Could you check a few things on this model? Use its own coordinates, in mm. Face numbers are marked on the shaded views. Give positions to 0.01 mm unless a question says otherwise; leave off trailing zeros. Order: outer loops, then holes, each group sorted by start corner. A loop starts at its lowest first (then second) coordinate and runs counter-clockwise, first axis right, second up. Notation, with made-up numbers: M 24,45.5 L 57,45.5 A23 ccw 57,79.5 Z; hole C -19,43 d9. An arc over 180 degrees is marked long. Answer in a Markdown table with one row per item. Add a question column.
```python
from build123d import *

# Parameters (mm, degrees)
F0_R     = 6.5
F1_DEPTH = 49.2
F2_DEPTH = 32
F3_DEPTH = 41.7


with BuildPart() as f1:
    # F0 (on Front) → F1 (new body)
    with BuildSketch(Plane.XZ):
        with BuildLine():
            Line((24.735266, 68.032924), (18.390851, 76.765262))
            ThreePointArc((18.390851, 76.765262), (-46.398298, 63.861779), (-78.691188, 6.231032))
            Line((-78.691188, 6.231032), (-72.346773, -2.501307))
            ThreePointArc((-72.346773, -2.501307), (-42.549774, 58.56474), (24.735266, 68.032924))
        make_face()
        with BuildLine():
            Line((37.798947, 50.052309), (24.735266, 68.032924))
            ThreePointArc((24.735266, 68.032924), (-42.549774, 58.56474), (-72.346773, -2.501307))
            Line((-72.346773, -2.501307), (-59.283092, -20.481921))
            Line((-59.283092, -20.481921), (-28.170116, 2.122979))
            ThreePointArc((-28.170116, 2.122979), (-16.604933, 22.85473), (6.685972, 27.447409))
            Line((6.685972, 27.447409), (37.798947, 50.052309))
        make_face()
        with Locations((-54.35288, 17.660321)):
            Circle(F0_R, mode=Mode.SUBTRACT)
        with Locations((0, 57.15)):
            Circle(F0_R, mode=Mode.SUBTRACT)
    extrude(amount=F1_DEPTH)

    # F0 (on Front) → F2 (join)
    with BuildSketch(Plane.XZ):
        with BuildLine():
            Line((18.390851, 76.765262), (-49.64947, 170.41473))
            ThreePointArc((-49.64947, 170.41473), (-104.331882, 143.600517), (-146.731509, 99.8805))
            Line((-146.731509, 99.8805), (-78.691188, 6.231032))
            ThreePointArc((-78.691188, 6.231032), (-46.398298, 63.861779), (18.390851, 76.765262))
        make_face()
    extrude(amount=F2_DEPTH)

    # F0 (on Front) → F3 (cut)
    with BuildSketch(Plane.XZ):
        with BuildLine():
            Line((37.798947, 50.052309), (24.735266, 68.032924))
            ThreePointArc((24.735266, 68.032924), (-42.549774, 58.56474), (-72.346773, -2.501307))
            Line((-72.346773, -2.501307), (-59.283092, -20.481921))
            Line((-59.283092, -20.481921), (-28.170116, 2.122979))
            ThreePointArc((-28.170116, 2.122979), (-16.604933, 22.85473), (6.685972, 27.447409))
            Line((6.685972, 27.447409), (37.798947, 50.052309))
        make_face()
        with Locations((-54.35288, 17.660321)):
            Circle(F0_R, mode=Mode.SUBTRACT)
        with Locations((0, 57.15)):
            Circle(F0_R, mode=Mode.SUBTRACT)
    extrude(amount=F3_DEPTH, mode=Mode.SUBTRACT)


solid = f1.part
```
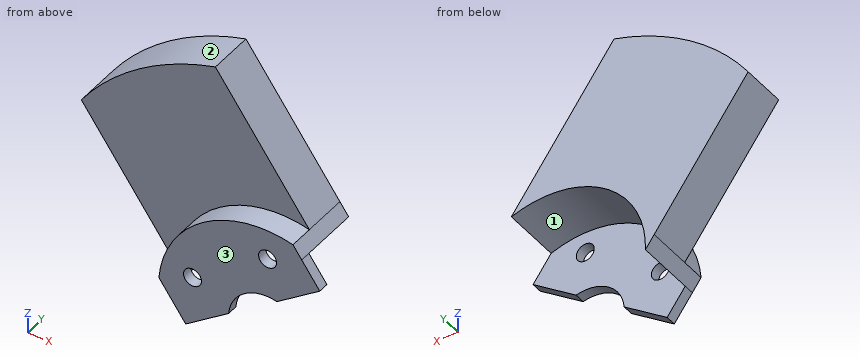
1. If I drill on line 1 along Y through (x, z) = (-79.5, 104.5); line 2 along Y through (x, z) = (-64, 0); line 3 along X through (y, z) = (-44, 57), over which ranges is the centre line in solid material (lowest first)? Write a range as [from, to].
2. Thinking about a two-plate mould opening in X: for the marked faces 1, 2 and 3, which applies, pulls with the +X half, pulls with the -X half, needs draft (parallel to the pull), parting line crosses it, or undercut?
3. Suppose I cut it at D-D on x = -11. List the corners of the cut face in (y, z) for me, plus the area to 3 significant figures.
4. Suppose I cut it at A-A on z = 57.15. List the corners of the cut face in (x, y) for me.
5. Suppose I cut it at B-B on x = -57. List the corners of the cut face in (y, z) for me, plus the area to 3 significant figures.
6. Will these pins go through, and if not, where does the flat tip stop? P1, Ø10, axis at x = -90.5, z = 108.5, coming from the -Y side; P2, Ø12, axis at x = -30.5, y = -8.5, coming from the -Z side; P3, Ø4, axis at x = -126, z = 66.5, coming from the -Y side; P4, Ø3, axis at x = 15, z = 35.5, coming from the +Y side.
7. Suppose I cut it at C-C on y = -28.5. List the corners of the cut face in (x, z) for me, plus the area to 3 significant figures.
Findings below:
| question | item | result |
|---|---|---|
| 1 | line 1 | [-32, 0] |
| 1 | line 2 | [-49.2, -41.7] |
| 1 | line 3 | [-54.61, -6.5], [6.5, 32.75] |
| 2 | face 1 | undercut |
| 2 | face 2 | pulls with the -X half |
| 2 | face 3 | needs draft |
| 3 | outline | M -49.2,26.02 L -41.7,26.02 L -41.7,71.55 L 0,71.55 L 0,117.22 L -32,117.22 L -32,78.17 L -49.2,78.17 Z |
| 3 | area | 1,920 mm2 |
| 4 | outline | M -115.69,-32 L -54.45,-32 L -54.45,-49.2 L -6.5,-49.2 L -6.5,-41.7 L -44.43,-41.7 L -44.43,0 L -115.69,0 Z; M 6.5,-49.2 L 32.64,-49.2 L 32.64,-41.7 L 6.5,-41.7 Z |
| 5 | outline | M -49.2,-18.82 L -41.7,-18.82 L -41.7,11.72 L -49.2,11.72 Z; M -49.2,23.6 L -41.7,23.6 L -41.7,44.62 L 0,44.62 L 0,168.1 L -32,168.1 L -32,54.61 L -49.2,54.61 Z |
| 5 | area | 4,510 mm2 |
| 6 | P1 | y = -32 |
| 6 | P2 | z = 62.51 |
| 6 | P3 | through |
| 6 | P4 | y = -41.7 |
| 7 | outline | M -146.73,99.88 L -72.35,-2.5 A72.39 cw 24.74,68.03 L -49.65,170.41 A177.5 ccw Z |
| 7 | area | 13,300 mm2 |
